Build history of the part. All positions in model axes, mm. Face numbers are marked on the shaded views. A direction names the side the tool comes from. Give positions to 0.01 mm unless a question says otherwise; leave off trailing zeros. Write each loop counter-clockwise with the first axis right and the second up, starting at its lowest first coordinate (ties: lowest second). Pieces come first, ordered by that corner, then holes. Notation, with made-up numbers: M 53,-30 L 111,-30 A30 ccw 111,1 Z; hole C 81,-36 d4. An arc over 180 degrees is marked long. Return JSON: item names as keys, results as strings. Group by question number.
Q1. Tool access for the marked faces 1 and 2: list every direction of +Z, -Z, +X, -X, +Y, -Y with a clear straight run to the whole face (end or side of a thin tool).
Q2. Band-saw the part on D-D, the plane y = -15. Give the cut face in (x, z), then the cut area to 3 significant figures.
Q3. Flat gauge pins, fed straight in: pin 1 Ø1.8 at (y, z) = (31.5, 7.5) entering from -X; pin 2 Ø3.5 at (x, y) = (22.72, -80.89) entering from -Z; pin 3 Ø1.3 at (x, z) = (86.5, 10.5) entering from +Y. Where does each tip first touch, or does it go through?
Q4. Band-saw the part on B-B, the plane x = -44.5. Give the cut face in (y, z).
Q5. Band-saw the part on A-A, the plane z = 7.75. Give the cut face in (x, y).
Q6. Wall check: probe 1 along X at (y, z) = (1.5, 4); probe 2 along Z at (x, y) = (23.5, -5); probe 3 along Y at (x, z) = (18, 11.5). Give the ranges that are in metal, low to high.
Q7. Band-saw the part on C-C, the plane y = 17.5. Give the cut face in (x, z), then the cut area to 3 significant figures.
from build123d import *

# Parameters (mm, degrees)
SKETCH1_W                                       = 170
SKETCH1_H                                       = 118
BOSS_EXTRUDE1_DEPTH                             = 2
EDGE_FLANGE4_STRIP_W                            = 11
EDGE_FLANGE4_STRIP_H                            = 2
EDGE_FLANGE4_STRIP_CUT_DEPTH                    = 170
EDGE_FLANGE4_DEPTH                              = 170
EDGE_FLANGE5_STRIP_W                            = 11
EDGE_FLANGE5_STRIP_H                            = 2
EDGE_FLANGE5_STRIP_CUT_DEPTH                    = 116.5
EDGE_FLANGE5_DEPTH                              = 116.5
EDGE_FLANGE6_STRIP_W                            = 11
EDGE_FLANGE6_STRIP_H                            = 2
EDGE_FLANGE6_STRIP_CUT_DEPTH                    = 116.5
EDGE_FLANGE6_DEPTH                              = 116.5
SKETCH26_W                                      = 18.240462441
SKETCH26_H                                      = 10
CUT_EXTRUDE2_DEPTH                              = 3.5
SKETCH27_W                                      = 23.960032842
SKETCH27_H                                      = 10
CUT_EXTRUDE3_DEPTH                              = 3.5
CSK_FOR_M3_FLAT_HEAD_MACHINE_SCREW2_D           = 3.2
CSK_FOR_M3_FLAT_HEAD_MACHINE_SCREW2_CSINK_D     = 6.3
CSK_FOR_M3_FLAT_HEAD_MACHINE_SCREW2_CSINK_ANGLE = 90
CUT_EXTRUDE4_REACH                              = 125.324
SKETCH32_R                                      = 7
CUT_EXTRUDE5_REACH                              = 125.324
SKETCH33_R                                      = 10.5
CUT_EXTRUDE6_START                              = -4
CUT_EXTRUDE6_OUTLINE_W                          = 1.43
CUT_EXTRUDE6_OUTLINE_H                          = 18
CUT_EXTRUDE6_OUTLINE_W_2                        = 1.43354479
CUT_EXTRUDE6_DEPTH                              = 4
CUT_EXTRUDE6_2_DEPTH                            = 0.5


# Read off the part's stored shape, not the designer's step: Cut-Extrude6
# Sheet-metal steps are written as plain solids
with BuildPart() as part:
    # Sketch1 → Boss-Extrude1 (new body)
    with BuildSketch(Plane.XY):
        with Locations((2.219863014, -26.886363636)):
            Rectangle(SKETCH1_W, SKETCH1_H)
    extrude(amount=BOSS_EXTRUDE1_DEPTH)

    # Edge-Flange4 strip (across the edge) → Edge-Flange4 strip cut (cut)
    with BuildSketch(Plane(origin=(87.219863014, 32.113636364, 2), x_dir=(0, -1, 0), z_dir=(-1, 0, 0))):
        with Locations((-4, -1)):
            Rectangle(EDGE_FLANGE4_STRIP_W, EDGE_FLANGE4_STRIP_H)
    extrude(amount=EDGE_FLANGE4_STRIP_CUT_DEPTH, mode=Mode.SUBTRACT)

    # Edge-Flange4 section (across the edge) → Edge-Flange4 (add)
    with BuildSketch(Plane(origin=(87.219863014, 32.113636364, 2), x_dir=(0, -1, 0), z_dir=(-1, 0, 0))):
        with BuildLine():
            Line((-2, 1.5), (-2, 13))
            Line((-2, 13), (0, 13))
            Line((0, 13), (0, 1.5))
            ThreePointArc((0, 1.5), (0.439339828, 0.439339828), (1.5, 0))
            Line((1.5, 0), (1.5, -2))
            ThreePointArc((1.5, -2), (-0.974873734, -0.974873734), (-2, 1.5))
        make_face()
    extrude(amount=EDGE_FLANGE4_DEPTH)

    # Edge-Flange5 strip (across the edge) → Edge-Flange5 strip cut (cut)
    with BuildSketch(Plane(origin=(-82.780136986, 30.613636364, 2), x_dir=(1, 0, 0), z_dir=(0, -1, 0))):
        with Locations((-2, -1)):
            Rectangle(EDGE_FLANGE5_STRIP_W, EDGE_FLANGE5_STRIP_H)
    extrude(amount=EDGE_FLANGE5_STRIP_CUT_DEPTH, mode=Mode.SUBTRACT)

    # Edge-Flange5 section (across the edge) → Edge-Flange5 (add)
    with BuildSketch(Plane(origin=(-82.780136986, 30.613636364, 2), x_dir=(1, 0, 0), z_dir=(0, -1, 0))):
        with BuildLine():
            Line((0, 1.5), (0, 13))
            Line((0, 13), (2, 13))
            Line((2, 13), (2, 1.5))
            ThreePointArc((2, 1.5), (2.439339828, 0.439339828), (3.5, 0))
            Line((3.5, 0), (3.5, -2))
            ThreePointArc((3.5, -2), (1.025126266, -0.974873734), (0, 1.5))
        make_face()
    extrude(amount=EDGE_FLANGE5_DEPTH)

    # Edge-Flange6 strip (across the edge) → Edge-Flange6 strip cut (cut)
    with BuildSketch(Plane(origin=(87.219863014, -85.886363636, 2), x_dir=(-1, 0, 0), z_dir=(0, 1, 0))):
        with Locations((-2, -1)):
            Rectangle(EDGE_FLANGE6_STRIP_W, EDGE_FLANGE6_STRIP_H)
    extrude(amount=EDGE_FLANGE6_STRIP_CUT_DEPTH, mode=Mode.SUBTRACT)

    # Edge-Flange6 section (across the edge) → Edge-Flange6 (add)
    with BuildSketch(Plane(origin=(87.219863014, -85.886363636, 2), x_dir=(-1, 0, 0), z_dir=(0, 1, 0))):
        with BuildLine():
            Line((0, 1.5), (0, 13))
            Line((0, 13), (2, 13))
            Line((2, 13), (2, 1.5))
            ThreePointArc((2, 1.5), (2.439339828, 0.439339828), (3.5, 0))
            Line((3.5, 0), (3.5, -2))
            ThreePointArc((3.5, -2), (1.025126266, -0.974873734), (0, 1.5))
        make_face()
    extrude(amount=EDGE_FLANGE6_DEPTH)

    # Sketch26 → Cut-Extrude2 (cut)
    with BuildSketch(Plane.ZY.offset(82.780136986)):
        with Locations((5.87976878, -80.886363636)):
            Rectangle(SKETCH26_W, SKETCH26_H)
    extrude(amount=-CUT_EXTRUDE2_DEPTH, mode=Mode.SUBTRACT)

    # Sketch27 → Cut-Extrude3 (cut)
    with BuildSketch(Plane(origin=(87.219863014, 0, 0), x_dir=(0, 0, -1), z_dir=(1, 0, 0))):
        with Locations((-3.019983579, -80.886363636)):
            Rectangle(SKETCH27_W, SKETCH27_H)
    extrude(amount=-CUT_EXTRUDE3_DEPTH, mode=Mode.SUBTRACT)

    # CSK for M3 Flat Head Machine Screw2 (through all)
    with Locations(Plane(origin=(0, 0, 0), x_dir=(-1, 0, 0), z_dir=(0, 0, -1))):
        with Locations((-72.719863014, -80.886363636), (-22.719863014, -80.886363636), (18.280136986, -80.886363636), (68.280136986, -80.886363636)):
            CounterSinkHole(CSK_FOR_M3_FLAT_HEAD_MACHINE_SCREW2_D / 2, CSK_FOR_M3_FLAT_HEAD_MACHINE_SCREW2_CSINK_D / 2, counter_sink_angle=CSK_FOR_M3_FLAT_HEAD_MACHINE_SCREW2_CSINK_ANGLE)

    # Sketch32 → Cut-Extrude4 (cut, up to next)
    with BuildSketch(Plane(origin=(0, 0, 0), x_dir=(-1, 0, 0), z_dir=(0, 0, -1)), mode=Mode.PRIVATE) as cut_extrude4_sk1:
        with Locations((-19.678120583, -12.276718373)):
            Circle(SKETCH32_R)
    cut_extrude4_tool1 = extrude(cut_extrude4_sk1.sketch, amount=-CUT_EXTRUDE4_REACH, mode=Mode.PRIVATE) & part.part
    add(cut_extrude4_tool1.solids().sort_by_distance((19.678121, -12.276718, 0))[0], mode=Mode.SUBTRACT)

    # Sketch33 → Cut-Extrude5 (cut, up to next)
    with BuildSketch(Plane(origin=(0, 0, 0), x_dir=(-1, 0, 0), z_dir=(0, 0, -1)), mode=Mode.PRIVATE) as cut_extrude5_sk1:
        with Locations((58.713568672, -59.876553933)):
            Circle(SKETCH33_R)
    cut_extrude5_tool1 = extrude(cut_extrude5_sk1.sketch, amount=-CUT_EXTRUDE5_REACH, mode=Mode.PRIVATE) & part.part
    add(cut_extrude5_tool1.solids().sort_by_distance((-58.713569, -59.876554, 0))[0], mode=Mode.SUBTRACT)

    # Cut-Extrude6 outline → Cut-Extrude6 (cut)
    with BuildSketch(Plane(origin=(0, 34.113636364, 0), x_dir=(1, 0, 0), z_dir=(0, 1, 0)).offset(CUT_EXTRUDE6_START)):
        with Locations((86.504863014, -8)):
            Rectangle(CUT_EXTRUDE6_OUTLINE_W, CUT_EXTRUDE6_OUTLINE_H)
        with Locations((-82.063364591, -8)):
            Rectangle(CUT_EXTRUDE6_OUTLINE_W_2, CUT_EXTRUDE6_OUTLINE_H)
    extrude(amount=CUT_EXTRUDE6_DEPTH, mode=Mode.SUBTRACT)

    # Cut-Extrude6 2 outline → Cut-Extrude6 2 (cut)
    with BuildSketch(Plane(origin=(0, 34.113636364, 0), x_dir=(1, 0, 0), z_dir=(0, 1, 0)).offset(CUT_EXTRUDE6_START)):
        Polygon((85.789863014, -17), (85.789863014, -0.677749125), (84.607005871, -2.290463911), (73.818191888, -17), align=None)
        Polygon((-81.346592196, -17), (-69.404507856, -17), (-80.165760648, -2.289351112), (-81.346592196, -0.675152595), align=None)
    extrude(amount=CUT_EXTRUDE6_2_DEPTH, mode=Mode.SUBTRACT)


solid = part.part
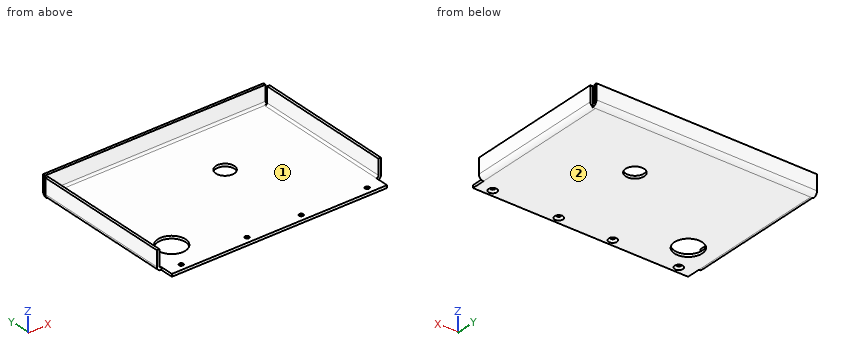
From the geometry:
{
 "1": {"face 1": "+Z, -Y", "face 2": "-Z, +X, -X, +Y, -Y"},
 "2": {"outline": "M -82.78,3.5 A3.5 ccw -79.28,0 L 13.23,0 L 13.23,2 L -79.28,2 A1.5 cw -80.78,3.5 L -80.78,15 L -82.78,15 Z; M 26.13,0 L 83.72,0 A3.5 ccw 87.22,3.5 L 87.22,15 L 85.22,15 L 85.22,3.5 A1.5 cw 83.72,2 L 26.13,2 Z", "area": "362 mm^2"},
 "3": {"pin 1": "stops at x = -81.35", "pin 2": "stops at z = 1.4", "pin 3": "stops at y = 30.11"},
 "4": {"outline": "M -85.89,0 L 30.61,0 A3.5 ccw 34.11,3.5 L 34.11,15 L 32.11,15 L 32.11,3.5 A1.5 cw 30.61,2 L -85.89,2 Z"},
 "5": {"outline": "M -82.78,-75.89 L -80.78,-75.89 L -80.78,30.11 L -82.78,30.11 Z; M -81.35,32.11 L 85.79,32.11 L 85.79,34.11 L -81.35,34.11 Z; M 85.22,-75.89 L 87.22,-75.89 L 87.22,30.11 L 85.22,30.11 Z"},
 "6": {"probe 1": "x = -82.78 to -80.78, 85.22 to 87.22", "probe 2": "z = 0 to 2", "probe 3": "y = 32.11 to 34.11"},
 "7": {"outline": "M -82.78,3.5 A3.5 ccw -79.28,0 L 83.72,0 A3.5 ccw 87.22,3.5 L 87.22,15 L 85.22,15 L 85.22,3.5 A1.5 cw 83.72,2 L -79.28,2 A1.5 cw -80.78,3.5 L -80.78,15 L -82.78,15 Z", "area": "388 mm^2"}
}
